Here's how the part is built. I have some questions about the finished solid (model axes, mm). A direction names the side the tool comes from. Round coordinates to 2 decimals unless told otherwise and drop trailing zeros. Order: outer loops, then holes, each group sorted by start corner. A loop starts at its lowest first (then second) coordinate and runs counter-clockwise, first axis right, second up. Notation, with made-up numbers: (-26, -21) -> (-3, -21) arc R24 ccw to (-3, 9) -> close; hole circle Ø9 at (33.25, 12). An arc over 180 degrees is marked (long way). Use a Markdown table: item, result. Add a question column.
(1) On a 3-axis mill with a long thin cutter (end or side, diameter ignored), from which of +Z, -Z, +X, -X, +Y, -Y can I reach the whole of each face in a straight line? I mean faces 1 (the face through (0, 0, 90)), 2 (the face through (93.84, 37.09, -0.79)), 3 (the face through (0, 0, -88)), 4 (the face through (-1, 19, -87.5)). Say none if no direction works.
(2) I want a section at C-C, the plane x = 0. Please give me the cut outline in (y, z), then the cut area to 3 significant figures.
(3) I want a section at D-D, the plane z = 0. Please give me the cut outline in (x, y), then the cut area to 3 significant figures.
(4) I'm going to push flat-ended pins straight in: P1, Ø7.5, axis at x = -116, y = 13.5, coming from the +Z side; P2, Ø24, axis at y = 17.5, z = -73, coming from the -X side; P3, Ø10.5, axis at x = -93.69, z = 93.05, coming from the +Y side. Where does each tip first touch, or does it pass through?
(5) If I drill on probe 1 along X at (y, z) = (14, 55); probe 2 along Y at (x, z) = (0, -95), over which ranges is the centre line in solid material (lowest first)?
(6) I want a section at A-A, the plane z = 40. Please give me the cut outline in (x, y), then the cut area to 3 significant figures.
(7) Thinking about a two-plate mould opening in Y: for faces 5 (the face through (94, -7, 0)), 6 (the face through (94, 45, 0)), 7 (the face through (-115, 16, 11.373)), 8 (the face through (-0.87, 9.71, 93.84)), which applies, pulls with the +Y half, pulls with the -Y half, needs draft (parallel to the pull), parting line crosses it, or undercut?
(8) I want a section at B-B, the plane y = 22. Give the number of separate pieces and of enclosed holes in the cut face, then the cut area to 3 significant figures.
from build123d import *

# Parameters (mm, degrees)
SKETCH1_W           = 200
SKETCH1_H           = 200
BOSS_EXTRUDE1_DEPTH = 30
SKETCH4_W           = 175
SKETCH4_H           = 175
CUT_EXTRUDE1_DEPTH  = 30
SKETCH7_R           = 4
CUT_EXTRUDE2_DEPTH  = 210
SKETCH10_W          = 6.040230253
SKETCH10_H          = 30
BOSS_EXTRUDE2_DEPTH = 20
SKETCH11_W          = 10
SKETCH11_H          = 30
BOSS_EXTRUDE3_DEPTH = 20
CUT_EXTRUDE3_START  = -231
SKETCH12_R          = 4
CUT_EXTRUDE3_DEPTH  = 231
SKETCH13_R          = 4
CUT_EXTRUDE5_DEPTH  = 231
SKETCH14_R          = 4
CUT_EXTRUDE6_DEPTH  = 250.5
SKETCH15_R          = 30
SKETCH15_R_2        = 22
BOSS_EXTRUDE5_DEPTH = 201
SKETCH17_R          = 22
CUT_EXTRUDE7_DEPTH  = 201
SKETCH21_W          = 9.5
SKETCH21_H          = 28.855904386
BOSS_EXTRUDE6_DEPTH = 26
SKETCH22_W          = 9.5
SKETCH22_H          = 6.040230253
CUT_EXTRUDE10_DEPTH = 49
SKETCH23_W          = 10.008922512
SKETCH23_H          = 28.855904386
BOSS_EXTRUDE7_DEPTH = 21
SKETCH24_W          = 9.5
SKETCH24_H          = 1.144095614
CUT_EXTRUDE11_DEPTH = 27
SKETCH26_W          = 0.50137975
SKETCH26_H          = 20.893624798
CUT_EXTRUDE12_DEPTH = 35
SKETCH27_R          = 49.192783102
CUT_EXTRUDE13_DEPTH = 175
SKETCH28_R          = 41.209023923
CUT_EXTRUDE14_DEPTH = 175


with BuildPart() as part:
    # Sketch1 → Boss-Extrude1 (new body)
    with BuildSketch(Plane(origin=(0, 0, 0), x_dir=(1, 0, 0), z_dir=(0, 1, 0))):
        Rectangle(SKETCH1_W, SKETCH1_H)
    extrude(amount=BOSS_EXTRUDE1_DEPTH)

    # Sketch4 → Cut-Extrude1 (cut)
    with BuildSketch(Plane(origin=(0, 30, 0), x_dir=(1, 0, 0), z_dir=(0, 1, 0))):
        Rectangle(SKETCH4_W, SKETCH4_H)
    extrude(amount=-CUT_EXTRUDE1_DEPTH, mode=Mode.SUBTRACT)

    # Sketch7 → Cut-Extrude2 (cut)
    with BuildSketch(Plane.ZY.offset(100)):
        with Locations((0, 15)):
            Circle(SKETCH7_R)
    extrude(amount=-CUT_EXTRUDE2_DEPTH, mode=Mode.SUBTRACT)

    # Sketch10 → Boss-Extrude2 (add)
    with BuildSketch(Plane.ZY.offset(100)):
        with Locations((-11.64671233, 15)):
            Rectangle(SKETCH10_W, SKETCH10_H)
    extrude(amount=BOSS_EXTRUDE2_DEPTH)

    # Sketch11 → Boss-Extrude3 (add)
    with BuildSketch(Plane.XY.offset(-8.626597203)):
        with Locations((-115, 15)):
            Rectangle(SKETCH11_W, SKETCH11_H)
    extrude(amount=BOSS_EXTRUDE3_DEPTH)

    # Sketch12 → Cut-Extrude3 (cut)
    with BuildSketch(Plane(origin=(100, 0, 0), x_dir=(0, 0, -1), z_dir=(1, 0, 0)).offset(CUT_EXTRUDE3_START)):
        with Locations(Location((0, 15, 0), (0, 0, 180))):
            Circle(SKETCH12_R)
    extrude(amount=CUT_EXTRUDE3_DEPTH, mode=Mode.SUBTRACT)

    # Sketch13 → Cut-Extrude5 (cut)
    with BuildSketch(Plane(origin=(0, 30, 0), x_dir=(1, 0, 0), z_dir=(0, 1, 0))):
        with Locations(Location((-93.69452155, -93.045501349, 0), (0, 0, 270))):
            Circle(SKETCH13_R)
    extrude(amount=-CUT_EXTRUDE5_DEPTH, mode=Mode.SUBTRACT)

    # Sketch14 → Cut-Extrude6 (cut)
    with BuildSketch(Plane.XY.offset(100)):
        with Locations((0, 13.614739596)):
            Circle(SKETCH14_R)
    extrude(amount=-CUT_EXTRUDE6_DEPTH, mode=Mode.SUBTRACT)

    # Sketch15 → Boss-Extrude5 (add)
    with BuildSketch(Plane(origin=(100, 0, 0), x_dir=(0, 0, -1), z_dir=(1, 0, 0))):
        with Locations((0, 15)):
            Circle(SKETCH15_R)
        with Locations((0, 15)):
            Circle(SKETCH15_R_2, mode=Mode.SUBTRACT)
    extrude(amount=-BOSS_EXTRUDE5_DEPTH)

    # Sketch17 → Cut-Extrude7 (cut)
    with BuildSketch(Plane(origin=(100, 0, 0), x_dir=(0, 0, -1), z_dir=(1, 0, 0))):
        with Locations((0.074377339, 15.100772812)):
            Circle(SKETCH17_R)
    extrude(amount=-CUT_EXTRUDE7_DEPTH, mode=Mode.SUBTRACT)


with BuildPart() as cut_extrude7_piece_1:
    # of the separate pieces the step leaves, piece 1, a body of its own (cut_extrude7_pieces)
    add(part.part.solids().sort_by_distance((-100, 0, -100))[0])



with BuildPart() as cut_extrude7_piece_2:
    # of the separate pieces the step leaves, piece 2, a body of its own (cut_extrude7_pieces)
    add(part.part.solids().sort_by_distance((-101, 0, -14.666827456))[0])

    # Sketch21 → Boss-Extrude6 (add)
    with BuildSketch(Plane(origin=(0, 0, -14.666827456), x_dir=(-1, 0, 0), z_dir=(0, 0, -1))):
        with Locations((115.25, 15.572047807)):
            Rectangle(SKETCH21_W, SKETCH21_H)
    extrude(amount=BOSS_EXTRUDE6_DEPTH)

    # Sketch22 → Cut-Extrude10 (cut)
    with BuildSketch(Plane(origin=(0, 30, 0), x_dir=(1, 0, 0), z_dir=(0, 1, 0))):
        with Locations((-105.75, 11.64671233)):
            Rectangle(SKETCH22_W, SKETCH22_H)
    extrude(amount=-CUT_EXTRUDE10_DEPTH, mode=Mode.SUBTRACT)


with BuildPart() as cut_extrude7_piece_1_1:
    add(cut_extrude7_piece_1.part)

    add(cut_extrude7_piece_2.part)  # Boss-Extrude7 merges Cut-Extrude7 piece 2
    # Sketch23 → Boss-Extrude7 (add)
    with BuildSketch(Plane(origin=(-110.5, 0, 0), x_dir=(0, 0, -1), z_dir=(1, 0, 0))):
        with Locations((35.6623662, 15.572047807)):
            Rectangle(SKETCH23_W, SKETCH23_H)
    extrude(amount=BOSS_EXTRUDE7_DEPTH)

    # Sketch24 → Cut-Extrude11 (cut)
    with BuildSketch(Plane(origin=(0, 0, -14.666827456), x_dir=(-1, 0, 0), z_dir=(0, 0, -1))):
        with Locations((115.25, 0.572047807)):
            Rectangle(SKETCH24_W, SKETCH24_H)
    extrude(amount=-CUT_EXTRUDE11_DEPTH, mode=Mode.SUBTRACT)

    # Sketch26 → Cut-Extrude12 (cut)
    with BuildSketch(Plane.XZ):
        with Locations((-110.249310125, 1.820215196)):
            Rectangle(SKETCH26_W, SKETCH26_H)
    extrude(amount=-CUT_EXTRUDE12_DEPTH, mode=Mode.SUBTRACT)

    # Sketch27 → Cut-Extrude13 (cut)
    with BuildSketch(Plane(origin=(-87.5, 0, 0), x_dir=(0, 0, -1), z_dir=(1, 0, 0))):
        with Locations((-31.916352411, 15.376133278)):
            Circle(SKETCH27_R)
    extrude(amount=CUT_EXTRUDE13_DEPTH, mode=Mode.SUBTRACT)

    # Sketch28 → Cut-Extrude14 (cut)
    with BuildSketch(Plane(origin=(-87.5, 0, 0), x_dir=(0, 0, -1), z_dir=(1, 0, 0))):
        with Locations((37.762434774, 15.494435184)):
            Circle(SKETCH28_R)
    extrude(amount=CUT_EXTRUDE14_DEPTH, mode=Mode.SUBTRACT)


solid = cut_extrude7_piece_1_1.part
Taken from the geometry:
| question | item | result |
|---|---|---|
| 1 | face 1 | +Z, +X, -X, -Y |
| 1 | face 2 | +X |
| 1 | face 3 | -Z, +X, -X, -Y |
| 1 | face 4 | +Y, -Y |
| 2 | outline | (-14.05, -7.51) arc R30 ccw to (-13.71, -8.69) arc R41.21 cw to (-13.16, -8.15) arc R49.19 cw to start; (0, -100) -> (9.61, -100) -> (9.61, -87.5) -> (0, -87.5) -> close; (0, 87.5) -> (9.61, 87.5) -> (9.61, 100) -> (0, 100) -> close; (17.61, -100) -> (30, -100) -> (30, -87.5) -> (17.61, -87.5) -> close; (17.61, 87.5) -> (30, 87.5) -> (30, 100) -> (17.61, 100) -> close |
| 2 | area | 550 mm2 |
| 3 | outline | (-120, 1.14) -> (-110.5, 1.14) -> (-110.5, 11) -> (-120, 11) -> close; (-120, 19) -> (-110.5, 19) -> (-110.5, 30) -> (-120, 30) -> close; (-101, -15) -> (-87.5, -15) -> (-87.5, -7) -> (-101, -7) -> close; (-101, 37.1) -> (-87.5, 37.1) -> (-87.5, 45) -> (-101, 45) -> close; (87.5, -15) -> (100, -15) -> (100, -7) -> (87.5, -7) -> close; (87.5, 37.1) -> (100, 37.1) -> (100, 45) -> (87.5, 45) -> close |
| 3 | area | 612 mm2 |
| 4 | P1 | stops at z = 11.37 |
| 4 | P2 | stops at x = -100 |
| 4 | P3 | stops at y = 30 |
| 5 | probe 1 | x = -100 to -87.5, 87.5 to 100 |
| 5 | probe 2 | y = 0 to 9.61, 17.61 to 30 |
| 6 | outline | (-100, 0) -> (-87.5, 0) -> (-87.5, 30) -> (-100, 30) -> close; (87.5, 0) -> (100, 0) -> (100, 30) -> (87.5, 30) -> close |
| 6 | area | 750 mm2 |
| 7 | face 5 | undercut |
| 7 | face 6 | pulls with the +Y half |
| 7 | face 7 | needs draft |
| 7 | face 8 | undercut |
| 8 | separate pieces | 2 |
| 8 | enclosed holes | 1 |
| 8 | area | 8,900 mm2 |
